Check sheet for the modelled part. Datum: model origin and axes. Units: mm. Give positions to 0.01 mm unless a question says otherwise; leave off trailing zeros. Order: outer loops, then holes, each group sorted by start corner. A loop starts at its lowest first (then second) coordinate and runs counter-clockwise, first axis right, second up.
Item 1: Sectioned sample at A-A on y = -17.5. Record the boundary of the cut face in (x, z).
Item 2: Sectioned sample at B-B on x = 32.9. Record the boundary of the cut face in (y, z).
Item 3: Material ranges on line 1 along Y through (x, z) = (32.9, 1.9); line 2 along Y through (x, z) = (2, 4.8); line 3 along X through (y, z) = (-2.25, 2.1), recorded low to high.
Item 4: Sectioned sample at C-C on z = 3.6. Record the boundary of the cut face in (x, y), and give its area (3 significant figures).
Item 5: Gauge pin test, flat end, axial feed: P1, Ø5, axis at x = 18, y = -5.5, coming from the -Z side. Record the tip position at first contact, or that the pin passes through.
from build123d import *

# Parameters (mm, degrees)
SKETCH1_W           = 5
SKETCH1_H           = 5
SKETCH1_R           = 1.25
BOSS_EXTRUDE1_DEPTH = 5


with BuildPart() as part:
    # Sketch1 → Boss-Extrude1 (new body)
    with BuildSketch(Plane.XY):
        Polygon((30.4, 0), (5, 0), (5, -5), (0, -5), (0, -15), (5, -15), (5, -20), (30.4, -20), (30.4, -15), (35.4, -15), (35.4, -5), (30.4, -5), align=None)
        with Locations((2.5, -2.5)):
            Rectangle(SKETCH1_W, SKETCH1_H)
        with Locations((2.5, -2.5)):
            Circle(SKETCH1_R, mode=Mode.SUBTRACT)
        with Locations((32.9, -2.5)):
            Rectangle(SKETCH1_W, SKETCH1_H)
        with Locations((32.9, -2.5)):
            Circle(SKETCH1_R, mode=Mode.SUBTRACT)
        with Locations((32.9, -17.5)):
            Rectangle(SKETCH1_W, SKETCH1_H)
        with Locations((32.9, -17.5)):
            Circle(SKETCH1_R, mode=Mode.SUBTRACT)
        with Locations((2.5, -17.5)):
            Rectangle(SKETCH1_W, SKETCH1_H)
        with Locations((2.5, -17.5)):
            Circle(SKETCH1_R, mode=Mode.SUBTRACT)
    extrude(amount=BOSS_EXTRUDE1_DEPTH)


solid = part.part
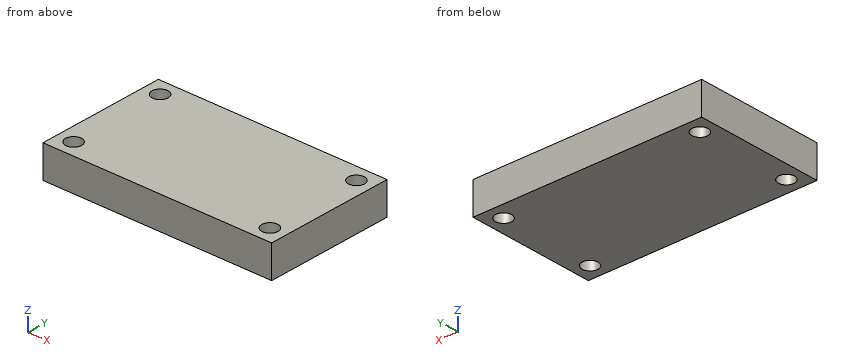
Report:
1. outline: (0, 0) - (1.25, 0) - (1.25, 5) - (0, 5) - close; (3.75, 0) - (31.65, 0) - (31.65, 5) - (3.75, 5) - close; (34.15, 0) - (35.4, 0) - (35.4, 5) - (34.15, 5) - close
2. outline: (-20, 0) - (-18.75, 0) - (-18.75, 5) - (-20, 5) - close; (-16.25, 0) - (-3.75, 0) - (-3.75, 5) - (-16.25, 5) - close; (-1.25, 0) - (0, 0) - (0, 5) - (-1.25, 5) - close
3. line 1: y = -20 to -18.75, -16.25 to -3.75, -1.25 to 0
3. line 2: y = -20 to -18.65, -16.35 to -3.65, -1.35 to 0
3. line 3: x = 0 to 1.28, 3.72 to 31.68, 34.12 to 35.4
4. outline: (0, -20) - (35.4, -20) - (35.4, 0) - (0, 0) - close; hole circle Ø2.5 at (2.5, -17.5); hole circle Ø2.5 at (2.5, -2.5); hole circle Ø2.5 at (32.9, -17.5); hole circle Ø2.5 at (32.9, -2.5)
4. area: 688 mm2
5. P1: stops at z = 0
